Geometry check sheet. Reference: drawing and pictorial views, mm from the part's lowest x, y, z. Give positions to 0.01 mm unless a question says otherwise; leave off trailing zeros. Write each loop counter-clockwise with the first axis right and the second up, starting at its lowest first coordinate (ties: lowest second). Pieces come first, ordered by that corner, then holes. Notation, with made-up numbers: (12, 43) -> (43, 43) arc R32 ccw to (43, 72) -> close; hole circle Ø9 at (30.5, -34). An arc over 180 degrees is marked (long way). Answer as CSV lines item,"result".
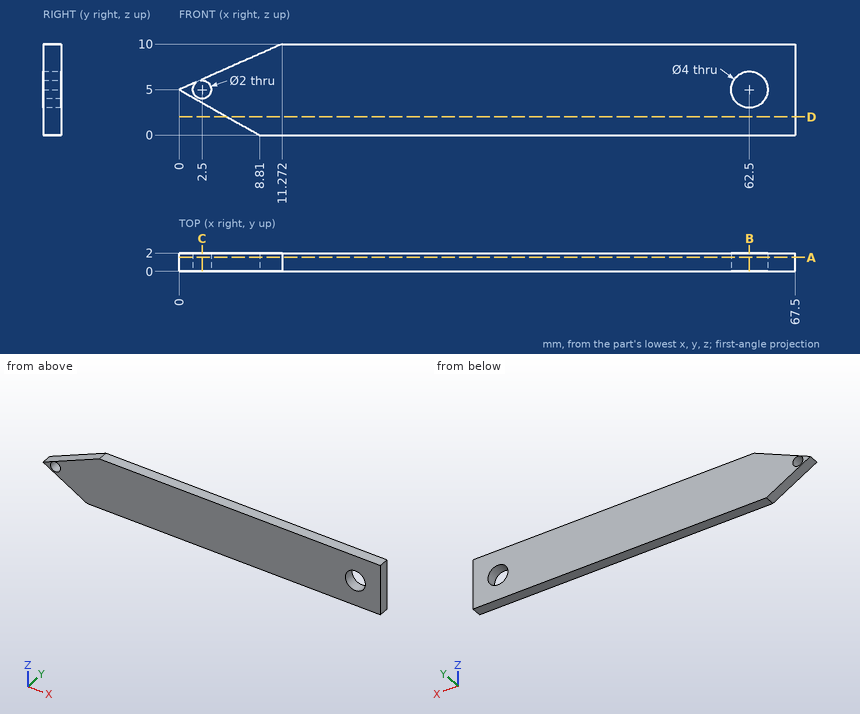
1) Section check A-A (y = 1.55). Record the boundary of the cut face in (x, z).
Reported:
outline,"(0, 5) -> (8.81, 0) -> (67.5, 0) -> (67.5, 10) -> (11.27, 10) -> close; hole circle Ø2 at (2.5, 5); hole circle Ø4 at (62.5, 5)"
2) Depth check by flat-ended pin: pin 1 (1.8 mm diameter, centred on x = 2.5, z = 5, fed in from -Y). Enter the tip coordinate at first touch or a pass-through.
Reported:
pin 1,"through"
3) Scan lines: line 1 along X through (y, z) = (0.9, 4.25) (1 decimal); line 2 along X through (y, z) = (1.3, 3.25) (1 decimal); line 3 along X through (y, z) = (1.1, 3.75) (1 decimal). Record each from-to range of solid material in increasing order.
Reported:
line 1,"1.3 to 1.8, 3.2 to 60.6, 64.4 to 67.5"
line 2,"3.1 to 61.5, 63.5 to 67.5"
line 3,"2.2 to 60.9, 64.1 to 67.5"
4) Section check C-C (x = 2.5). Record the boundary of the cut face in (y, z).
Reported:
outline,"(0, 3.58) -> (2, 3.58) -> (2, 4) -> (0, 4) -> close; (0, 6) -> (2, 6) -> (2, 6.11) -> (0, 6.11) -> close"
5) Section check D-D (z = 2). Record the boundary of the cut face in (x, y) (1 decimal).
Reported:
outline,"(5.3, 0) -> (67.5, 0) -> (67.5, 2) -> (5.3, 2) -> close"
6) Section check B-B (x = 62.5). Record the boundary of the cut face in (y, z), and give its area (3 significant figures).
Reported:
outline,"(0, 0) -> (2, 0) -> (2, 3) -> (0, 3) -> close; (0, 7) -> (2, 7) -> (2, 10) -> (0, 10) -> close"
area,"12.0 mm²"
